Autodesk Inventor part; units mm, degrees
ref_plane "YZ Plane" through (0, 0, 0) normal (1, 0, 0) x (0, 1, 0)
ref_plane "XZ Plane" through (0, 0, 0) normal (0, 1, 0) x (-1, 0, 0)
ref_plane "XY Plane" through (0, 0, 0) normal (0, 0, 1) x (1, 0, 0)
sketch "Sketch1" plane through (0, 0, 0) normal (0, 1, 0) x (-1, 0, 0)
  circle A0 centre (0, 0) radius 2
  line L0 (0, 0) -> (0, -10)
  circle A1 centre (0, -10) radius 2
  line L1 (0, 0) -> (4, 0)
  line L2 (4, 0) -> (4, 5)
  line L3 (4, 5) -> (0, 5)
  line L4 (0, 5) -> (0, 0)
  line L5 (0, -10) -> (-4, -10)
  line L6 (-4, -10) -> (-4, -15)
  line L7 (-4, -15) -> (0, -15)
  line L8 (0, -15) -> (0, -10)
  line L9 (4, 5) -> (-4, 5)
  line L10 (-4, 5) -> (-4, -15)
  line L11 (-4, -15) -> (4, -15)
  line L12 (4, -15) -> (4, 5)
  line L13 (4, -15) -> (-4, -15)
  line L14 (-4, -15) -> (-4, -23)
  line L15 (-4, -23) -> (4, -23)
  line L16 (4, -23) -> (4, -15)
  line L17 (0, -10) -> (0, -85)
  line L18 (0, -85) -> (10, -85)
  circle A2 centre (0, -170) radius 2
  line L19 (0, -170) -> (0, -160)
  circle A3 centre (0, -160) radius 2
  line L20 (0, -170) -> (4, -170)
  line L21 (4, -170) -> (4, -175)
  line L22 (4, -175) -> (0, -175)
  line L23 (0, -175) -> (0, -170)
  line L24 (0, -160) -> (-4, -160)
  line L25 (-4, -160) -> (-4, -155)
  line L26 (-4, -155) -> (0, -155)
  line L27 (0, -155) -> (0, -160)
  line L28 (4, -175) -> (-4, -175)
  line L29 (-4, -175) -> (-4, -155)
  line L30 (-4, -155) -> (4, -155)
  line L31 (4, -155) -> (4, -175)
  line L32 (4, -155) -> (-4, -155)
  line L33 (-4, -155) -> (-4, -147)
  line L34 (-4, -147) -> (4, -147)
  line L35 (4, -147) -> (4, -155)
  dimension "d0" = 4
  dimension "d1" = 10
  dimension "d2" = 4
  dimension "d3" = 4
  dimension "d4" = 5
  dimension "d5" = 4
  dimension "d6" = 5
  dimension "d7" = 8
  dimension "d8" = 75
  dimension "d9" = 10
extrude "Extrusion1" add sketch "Sketch1" along normal blind 4 contours L1 L12 L11 L8 A1 L0 A0 | A0 L4 L3 L2 L1 | A0 L0 A1 L5 L10 L9 L4 | L16 L15 L17 L11 | A1 L8 L7 L6 L5 | L17 L15 L14 L7 | L20 L21 L22 L23 A2 | A2 L19 A3 L27 L30 L31 L20 | A2 L23 L28 L29 L24 A3 L19 | L30 L26 L33 L34 L35 | L24 L25 L26 L27 A3
sketch "Sketch2" plane through (0, 0, 0) normal (0, -1, 0) x (1, 0, 0)
  line L0 (4, -23) -> (-4, -23)
  line L1 (4, 5) -> (4, -23)
  line L2 (-4, -23) -> (4, -23)
  line L3 (4, -23) -> (4, -16)
  line L4 (4, -16) -> (-4, -16)
  line L5 (-4, -16) -> (-4, -23)
  line L6 (-4, -147) -> (4, -147)
  line L7 (-4, -147) -> (4, -147)
  line L8 (4, -147) -> (4, -154)
  line L9 (4, -154) -> (-4, -154)
  line L10 (-4, -154) -> (-4, -147)
  point P0 (0, 0)
  dimension "d12" = 7
  dimension "d13" = 7
extrude "Extrusion2" add sketch "Sketch2" along normal blind 32
sketch "Sketch3" plane through (0, -32, 0) normal (0, -1, 0) x (1, 0, 0)
  line L0 (4, -154) -> (4, -147)
  line L1 (-4, -16) -> (-4, -23)
  line L2 (4, -154) -> (-4, -154)
  line L3 (-4, -154) -> (-4, -16)
  line L4 (-4, -16) -> (4, -16)
  line L5 (4, -16) -> (4, -154)
  point P0 (0, 0)
extrude "Extrusion3" add sketch "Sketch3" against normal blind 8
sketch "Sketch4" plane through (0, 4, 0) normal (0, 1, 0) x (1, 0, 0)
  line L0 (4, 23) -> (4, 147)
  line L1 (4, 147) -> (-4, 147)
  line L2 (-4, 147) -> (-4, 152)
  line L3 (-4, 152) -> (4, 152)
  line L4 (4, 152) -> (4, 147)
  line L5 (4, 23) -> (-4, 23)
  line L6 (4, 23) -> (-4, 23)
  line L7 (-4, 23) -> (-4, 18)
  line L8 (-4, 18) -> (4, 18)
  line L9 (4, 18) -> (4, 23)
  line L10 (-4, 18) -> (4, 18)
  line L11 (4, 18) -> (4, 152)
  line L12 (4, 152) -> (-4, 152)
  line L13 (-4, 152) -> (-4, 18)
  point P0 (0, 0)
  point P1 (-4, 23)
  dimension "d18" = 8
  dimension "d19" = 5
  dimension "d20" = 8
  dimension "d21" = 5
extrude "Extrusion4" add sketch "Sketch4" along normal blind 4
sketch "Sketch5" plane through (0, -24, 0) normal (0, 1, 0) x (1, 0, 0)
  line L0 (4, 23) -> (-4, 23)
  line L1 (4, 23) -> (4, 147)
  line L2 (4, 23) -> (4, 147)
  line L3 (4, 85) -> (0, 85)
  line L4 (-4, 65) -> (4, 65)
  line L5 (4, 65) -> (4, 105)
  line L6 (4, 105) -> (-4, 105)
  line L7 (-4, 105) -> (-4, 65)
  line L8 (-4, 65) -> (4, 105) construction
  line L9 (4, 65) -> (-4, 105) construction
  point P0 (0, 0)
  point P1 (4, 65)
  point P2 (4, 105)
  dimension "d24" = 40
extrude "Extrusion5" add sketch "Sketch5" along normal up to surface (28 mm away)
fillet "Fillet1" radius 2 4 edges at (0, 4, -23) (0, 8, -18) (0, 8, -152) (0, 4, -147)
sketch "Sketch6" plane through (4, 0, 5) normal (1, 0, 0) x (0, 0, -1)
  point P0 (5, 0)
sketch "Sketch7" plane through (0, 8, 0) normal (0, 1, 0) x (1, 0, 0)
  line L0 (-4, 150) -> (4, 150)
  line L1 (4, 150) -> (4, 130)
  line L2 (4, 154) -> (4, 16)
  line L3 (4, 20) -> (-4, 20)
  line L4 (4, 20) -> (4, 40)
  line L5 (4, 130) -> (14, 130)
  line L6 (14, 130) -> (14, 120)
  line L7 (14, 120) -> (4, 120)
  line L8 (4, 120) -> (4, 130)
  line L9 (14, 130) -> (4, 130)
  line L10 (4, 130) -> (4, 140)
  line L11 (4, 140) -> (14, 140)
  line L12 (14, 140) -> (14, 130)
  line L13 (4, 40) -> (14, 40)
  line L14 (14, 40) -> (14, 50)
  line L15 (14, 50) -> (4, 50)
  line L16 (4, 50) -> (4, 40)
  line L17 (4, 40) -> (14, 40)
  line L18 (14, 40) -> (14, 30)
  line L19 (14, 30) -> (4, 30)
  line L20 (4, 30) -> (4, 40)
  line L21 (9, 40) -> (9, 45)
  line L22 (9, 40) -> (9, 35)
  circle A0 centre (9, 45) radius 1.5
  circle A1 centre (9, 35) radius 1.5
  line L23 (9, 130) -> (9, 135)
  line L24 (9, 130) -> (9, 125)
  circle A2 centre (9, 135) radius 1.5
  circle A3 centre (9, 125) radius 1.5
  point P0 (0, 0)
  dimension "d28" = 20
  dimension "d29" = 20
  dimension "d30" = 10
  dimension "d31" = 10
  dimension "d32" = 10
  dimension "d33" = 10
  dimension "d34" = 10
  dimension "d35" = 3
  dimension "d36" = 3
  dimension "d37" = 5
  dimension "d38" = 3
  dimension "d39" = 3
extrude "Extrusion6" add sketch "Sketch7" against normal blind 3
fillet "Fillet2" radius 5 8 edges at (4, 6.5, -120) (14, 6.5, -120) (4, 6.5, -140) (14, 6.5, -140) (4, 6.5, -30) (14, 6.5, -30) (14, 6.5, -50) (4, 6.5, -50)
properties part number "side_wall2"
For this review, take the finished solid that the model builds, in its own axes (mm). A direction names the side the tool comes from. Coordinates: 2 decimals unless noted, no trailing zeros. Order: outer loops, then holes, each group sorted by start corner. A loop starts at its lowest first (then second) coordinate and runs counter-clockwise, first axis right, second up. Notation, with made-up numbers: (43, 18) -> (91, 18) arc R26 cw to (91, 44) -> close; hole circle Ø9 at (77.5, 20.25). An arc over 180 degrees is marked (long way). Use CSV: the item, a comma, the result in double quotes. Start each with the question number.
Item 1: Insertion check: pin 1 (4 mm diameter, centred on x = 0.5, y = -16, fed in from +Z); pin 2 (4 mm diameter, centred on x = -0.5, z = -163.5, fed in from -Y); pin 3 (2.5 mm diameter, centred on x = 2, z = -165, fed in from +Y). Each pin has a flat end and moves straight along its axis. Give the tip position at first contact, or say it passes through.
Item 2: Wall thickness on probe 1 along Z at (x, y) = (9, 7.35); probe 2 along Z at (x, y) = (-2.5, -21); probe 3 along X at (y, z) = (2.65, 0): over which ranges is each line inside the solid? List them lowest first.
Item 3: We need section D-D, the plane x = 0. Give the number of separate pieces and of enclosed holes in the cut face, then the cut area to 3 significant figures.
Item 4: We need section C-C, the plane y = -19. Give the boundary of the cut face in (x, z), then the cut area to 3 significant figures.
Item 5: Draft analysis for pull direction Z (two halves, no side actions). For faces 4 (the face through (5, 6, -118)), 5 (the face through (0, 4, -45)), 6 (the face through (0, 2, -175)), 7 (the face through (0, -32, -84)), state which applies: pulls with the +Z half, pulls with the -Z half, needs draft (parallel to the pull), parting line crosses it, or undercut.
Item 6: We need section A-A, the plane z = 0. Give the boundary of the cut face in (x, y), then the cut area to 3 significant figures.
Item 7: For faces 1 (the face through (0, 4, -163)), 2 (the face through (6, 6, -51)), 3 (the face through (0, -11, -147)), list the 3-axis set-ups (+Z, -Z, +X, -X, +Y, -Y) from which the entire face can be reached by the end or side of a thin tool; tool diameter is ignored.
Item 8: We need section B-B, the plane x = 12.25. Give the boundary of the cut face in (y, z).
Derived:
1,pin 1,"stops at z = -16"
1,pin 2,"stops at y = 0"
1,pin 3,"stops at y = 4"
2,probe 1,"z = -140 to -136.5, -133.5 to -126.5, -123.5 to -120, -50 to -46.5, -43.5 to -36.5, -33.5 to -30"
2,probe 2,"z = -154 to -147, -105 to -65, -23 to -16"
2,probe 3,"x = -4 to -2, 2 to 4"
3,separate pieces,"5"
3,enclosed holes,"2"
3,area,"3,260 mm^2"
4,outline,"(-4, -154) -> (4, -154) -> (4, -147) -> (-4, -147) -> close; (-4, -105) -> (4, -105) -> (4, -65) -> (-4, -65) -> close; (-4, -23) -> (4, -23) -> (4, -16) -> (-4, -16) -> close"
4,area,"432 mm^2"
5,face 4,"undercut"
5,face 5,"undercut"
5,face 6,"pulls with the -Z half"
5,face 7,"needs draft"
6,outline,"(-4, 0) -> (-2, 0) -> (-2, 4) -> (-4, 4) -> close; (2, 0) -> (4, 0) -> (4, 4) -> (2, 4) -> close"
6,area,"16.0 mm^2"
7,face 1,"-Z, +X, -X, +Y"
7,face 2,"+X, +Y, -Y"
7,face 3,"+X, -X"
8,outline,"(5, -138.8) -> (8, -138.8) -> (8, -121.2) -> (5, -121.2) -> close; (5, -48.8) -> (8, -48.8) -> (8, -31.2) -> (5, -31.2) -> close"
